Design review of the part built by this model. Coordinates are the model's own, in mm. Face numbers are marked on the shaded views. Coordinates: 2 decimals unless noted, no trailing zeros. Order: outer loops, then holes, each group sorted by start corner. A loop starts at its lowest first (then second) coordinate and runs counter-clockwise, first axis right, second up. Notation, with made-up numbers: (69.5, 20) -> (85.5, 20) arc R11 cw to (85.5, 33) -> close; hole circle Ø7 at (56, 66). An arc over 180 degrees is marked (long way). Use a Markdown table: item, result. Add a question column.
Q1. Wall thickness on probe 1 along Z at (x, y) = (-280, -83.5); probe 2 along Z at (x, y) = (-290, -81.25); probe 3 along X at (y, z) = (-85, 25.5) (3 decimals): over which ranges is each line inside the solid? List them lowest first.
Q2. The part is to be moulded in two halves that separate along Z. For the marked faces 1 and 2, say which applies: pulls with the +Z half, pulls with the -Z half, needs draft (parallel to the pull), parting line crosses it, or undercut.
Q3. Add section B-B (x = -275.57). State the section outline as (y, z) points.
Q4. Add section C-C (z = 81.5). State the section outline as (x, y) points (3 decimals), then the cut area to 3 significant figures.
Q5. Add section A-A (x = -290.57). State the section outline as (y, z) points.
Q6. Insertion check: pin 1 (10 mm diameter, centred on x = -294.5, z = 21.5, fed in from +Y); pin 2 (17 mm diameter, centred on x = -253.55, z = 28.505, fed in from -Y); pin 3 (1 mm diameter, centred on x = -291, y = -80, fed in from -Z); pin 4 (3 mm diameter, centred on x = -258.5, y = -82, fed in from -Z). Each pin has a flat end and moves straight along its axis. Give the tip position at first contact, or say it passes through.
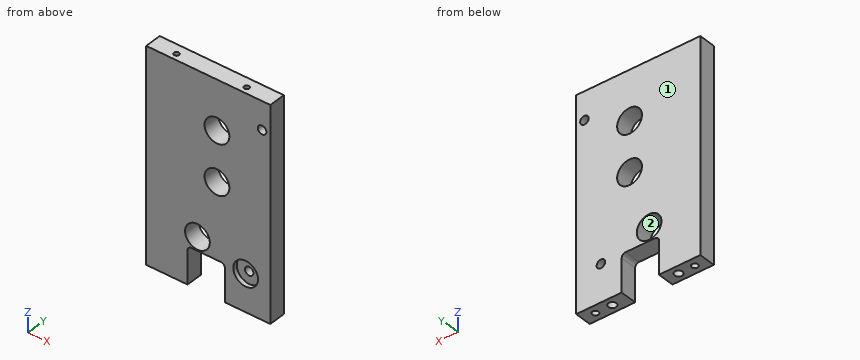
from build123d import *

# Parameters (mm, degrees)
SKETCH1_W           = 95.25
SKETCH1_H           = 12.8
BOSS_EXTRUDE1_DEPTH = 161.88
SKETCH1_3_R         = 3.1
CUT_EXTRUDE1_DEPTH  = 20.2
SKETCH1_4_R         = 2.395
CUT_EXTRUDE2_DEPTH  = 21.5
CUT_EXTRUDE3_REACH  = 14.8
SKETCH2_R           = 9.525
SKETCH2_R_2         = 3.265
SKETCH3_R           = 3.265
SKETCH3_R_2         = 9.525
CUT_EXTRUDE4_DEPTH  = 3.32
CUT_EXTRUDE5_START  = -17.25
SKETCH4_R           = 1.965
CUT_EXTRUDE5_DEPTH  = 17.25
SKETCH6_R           = 9.5
CUT_EXTRUDE6_DEPTH  = 13.8000001


with BuildPart() as part:
    # Sketch1 → Boss-Extrude1 (new body)
    with BuildSketch(Plane.XY):
        with Locations((-282.25, -82.5)):
            Rectangle(SKETCH1_W, SKETCH1_H)
    extrude(amount=BOSS_EXTRUDE1_DEPTH)

    # Sketch1<3> → Cut-Extrude1 (cut)
    with BuildSketch(Plane.XY):
        with Locations((-308, -82.5)):
            Circle(SKETCH1_3_R)
        with Locations((-257.2, -82.5)):
            Circle(SKETCH1_3_R)
    extrude(amount=CUT_EXTRUDE1_DEPTH, mode=Mode.SUBTRACT)

    # Sketch1<4> → Cut-Extrude2 (cut)
    with BuildSketch(Plane.XY):
        with Locations((-320.5, -82.5)):
            Circle(SKETCH1_4_R)
        with Locations((-244.2, -82.5)):
            Circle(SKETCH1_4_R)
    extrude(amount=CUT_EXTRUDE2_DEPTH, mode=Mode.SUBTRACT)

    # Sketch2 → Cut-Extrude3 (cut, up to next)
    with BuildSketch(Plane(origin=(0, -76.1, 0), x_dir=(-1, 0, 0), z_dir=(0, 1, 0)), mode=Mode.PRIVATE) as cut_extrude3_sk1:
        with Locations((275.57, 86.105)):
            Circle(SKETCH2_R)
    cut_extrude3_tool1 = extrude(cut_extrude3_sk1.sketch, amount=-CUT_EXTRUDE3_REACH, mode=Mode.PRIVATE) & part.part
    add(cut_extrude3_tool1.solids().sort_by_distance((-275.57, -76.1, 86.105))[0], mode=Mode.SUBTRACT)
    # Sketch2 → Cut-Extrude3 (cut, up to next)
    with BuildSketch(Plane(origin=(0, -76.1, 0), x_dir=(-1, 0, 0), z_dir=(0, 1, 0)), mode=Mode.PRIVATE) as cut_extrude3_sk2:
        with Locations((275.57, 124.135)):
            Circle(SKETCH2_R)
    cut_extrude3_tool2 = extrude(cut_extrude3_sk2.sketch, amount=-CUT_EXTRUDE3_REACH, mode=Mode.PRIVATE) & part.part
    add(cut_extrude3_tool2.solids().sort_by_distance((-275.57, -76.1, 124.135))[0], mode=Mode.SUBTRACT)
    # Sketch2 → Cut-Extrude3 (cut, up to next)
    with BuildSketch(Plane(origin=(0, -76.1, 0), x_dir=(-1, 0, 0), z_dir=(0, 1, 0)), mode=Mode.PRIVATE) as cut_extrude3_sk3:
        with Locations((253.55, 28.505)):
            Circle(SKETCH2_R_2)
    cut_extrude3_tool3 = extrude(cut_extrude3_sk3.sketch, amount=-CUT_EXTRUDE3_REACH, mode=Mode.PRIVATE) & part.part
    add(cut_extrude3_tool3.solids().sort_by_distance((-253.55, -76.1, 28.505))[0], mode=Mode.SUBTRACT)
    # Sketch2 → Cut-Extrude3 (cut, up to next)
    with BuildSketch(Plane(origin=(0, -76.1, 0), x_dir=(-1, 0, 0), z_dir=(0, 1, 0)), mode=Mode.PRIVATE) as cut_extrude3_sk4:
        with Locations((240.925, 140.49)):
            Circle(SKETCH2_R_2)
    cut_extrude3_tool4 = extrude(cut_extrude3_sk4.sketch, amount=-CUT_EXTRUDE3_REACH, mode=Mode.PRIVATE) & part.part
    add(cut_extrude3_tool4.solids().sort_by_distance((-240.925, -76.1, 140.49))[0], mode=Mode.SUBTRACT)
    # Sketch2 → Cut-Extrude3 (cut, up to next)
    with BuildSketch(Plane(origin=(0, -76.1, 0), x_dir=(-1, 0, 0), z_dir=(0, 1, 0)), mode=Mode.PRIVATE) as cut_extrude3_sk5:
        with BuildLine():
            Line((269.505, 25.4), (269.505, 0))
            Line((269.505, 0), (298.155, 0))
            Line((298.155, 0), (298.155, 25.4))
            ThreePointArc((298.155, 25.4), (297.276320344, 27.521320344), (295.155, 28.4))
            Line((295.155, 28.4), (272.505, 28.4))
            ThreePointArc((272.505, 28.4), (270.383679656, 27.521320344), (269.505, 25.4))
        make_face()
    cut_extrude3_tool5 = extrude(cut_extrude3_sk5.sketch, amount=-CUT_EXTRUDE3_REACH, mode=Mode.PRIVATE) & part.part
    add(cut_extrude3_tool5.solids().sort_by_distance((-283.83, -76.1, 14.135461))[0], mode=Mode.SUBTRACT)

    # Sketch3 → Cut-Extrude4 (cut)
    with BuildSketch(Plane.XZ.offset(88.9)):
        with Locations((-240.925, 140.49)):
            Circle(SKETCH3_R)
        with Locations((-253.55, 28.505)):
            Circle(SKETCH3_R_2)
    extrude(amount=-CUT_EXTRUDE4_DEPTH, mode=Mode.SUBTRACT)

    # Sketch4 → Cut-Extrude5 (cut)
    with BuildSketch(Plane.XY.offset(161.88).offset(CUT_EXTRUDE5_START)):
        with Locations((-256.825, -83.83)):
            Circle(SKETCH4_R)
        with Locations((-310.715, -83.83)):
            Circle(SKETCH4_R)
    extrude(amount=CUT_EXTRUDE5_DEPTH, mode=Mode.SUBTRACT)

    # Sketch6 → Cut-Extrude6 (cut, through all)
    with BuildSketch(Plane(origin=(0, -76.1, 0), x_dir=(-1, 0, 0), z_dir=(0, 1, 0))):
        with Locations((290.57, 38.77)):
            Circle(SKETCH6_R)
    extrude(amount=-CUT_EXTRUDE6_DEPTH, mode=Mode.SUBTRACT)


solid = part.part
Established:
| question | item | result |
|---|---|---|
| 1 | probe 1 | 28.4 to 77.67, 94.54 to 115.7, 132.57 to 161.88 |
| 1 | probe 2 | 28.4 to 29.29, 48.25 to 161.88 |
| 1 | probe 3 | -329.875 to -298.153, -269.507 to -254.827, -252.273 to -234.625 |
| 2 | face 1 | needs draft |
| 2 | face 2 | undercut |
| 3 | outline | (-88.9, 28.4) -> (-76.1, 28.4) -> (-76.1, 76.58) -> (-88.9, 76.58) -> close; (-88.9, 95.63) -> (-76.1, 95.63) -> (-76.1, 114.61) -> (-88.9, 114.61) -> close; (-88.9, 133.66) -> (-76.1, 133.66) -> (-76.1, 161.88) -> (-88.9, 161.88) -> close |
| 4 | outline | (-329.875, -88.9) -> (-283.908, -88.9) -> (-283.908, -76.1) -> (-329.875, -76.1) -> close; (-267.232, -88.9) -> (-234.625, -88.9) -> (-234.625, -76.1) -> (-267.232, -76.1) -> close |
| 4 | area | 1,010 mm^2 |
| 5 | outline | (-88.9, 28.4) -> (-76.1, 28.4) -> (-76.1, 29.27) -> (-88.9, 29.27) -> close; (-88.9, 48.27) -> (-76.1, 48.27) -> (-76.1, 161.88) -> (-88.9, 161.88) -> close |
| 6 | pin 1 | y = -76.1 |
| 6 | pin 2 | y = -85.58 |
| 6 | pin 3 | z = 28.4 |
| 6 | pin 4 | z = 20.2 |
